Verification items for the finished model (mm, model axes). A direction names the side the tool comes from. Coordinates: 2 decimals unless noted, no trailing zeros. Loops run counter-clockwise (first coordinate to the right, second up) from the corner with the lowest first, then second, coordinate; pieces in that order, holes last. Notation, with made-up numbers: (82, 31.25) - (126, 31.25) arc R10 cw to (126, 35.25) - close; hole circle Ø4 at (-21.5, -19). An arc over 180 degrees is marked (long way). Answer as CSV lines item,"result". Start each with the question number.
1. Gauge pin test, flat ends, axial feed: P1, Ø3, axis at x = 0, z = 15, coming from the +Y side; P2, Ø4, axis at y = 4, z = 26.5, coming from the -X side; P3, Ø4, axis at x = 0, z = 5, coming from the +Y side. Record the tip position at first contact, or that the pin passes through.
2. Release check for a two-part mould opening along Z. For faces 1 (the flat face through (-0.1, 0.7, 30)), 2 (the flat face through (-0.1, 0.7, 0)), 3 (the flat face through (2.04, 1, 14.79)), 4 (the cylindrical face through (-0.24, 0.01, 13.14)) record: pulls with the +Z half, pulls with the -Z half, needs draft (parallel to the pull), parting line crosses it, or undercut.
3. Cross-section at C-C (x = 4). Enter the section's corners in (y, z) (3 decimals), plus the area to 3 significant figures.
4. Cross-section at B-B (y = 7.5). Enter the section's corners in (x, z).
5. Cross-section at A-A (z = 25). Enter the section's corners in (x, y), plus the area to 3 significant figures.
6. Material ranges on line 1 (Z direction, x = 3.65, y = 4) (3 decimals); line 2 (X direction, y = 3, z = 9); line 3 (Y direction, x = 4, z = 25), recorded low to high. Write a range as [from, to].
7. Cross-section at D-D (y = 4.75). State how many separate pieces and enclosed holes the cut face has, plus the area to 3 significant figures.
8. Set-up check for faces 5 (the flat face through (3, 7, 15)), 6 (the flat face through (-5, 1.8, 14.8)): record each of +Z, -Z, +X, -X, +Y, -Y from which the full face is reachable in a straight line by a thin tool's end or side.
```python
from build123d import *

# Parameters (mm, degrees)
BOSS_EXTRUDE1_DEPTH     = 30
SKETCH2_R               = 1.75
SKETCH2_R_2             = 2
SKETCH2_R_3             = 1.875
CUT_EXTRUDE2_DEPTH      = 9
CUT_EXTRUDE2_DEPTH_BACK = 3
SKETCH3_R               = 1.75
SKETCH3_R_2             = 1.875
SKETCH3_R_3             = 2
CUT_EXTRUDE3_DEPTH      = 10


with BuildPart() as part:
    # Sketch1 → Boss-Extrude1 (new body)
    with BuildSketch(Plane.XY):
        Polygon((3, 1), (-3, 1), (-3, 9), (-5, 9), (-5, -1), (5, -1), (5, 9), (3, 9), align=None)
    extrude(amount=BOSS_EXTRUDE1_DEPTH)

    # Sketch2 → Cut-Extrude2 (cut, two sides)
    with BuildSketch(Plane(origin=(-3, 0, 0), x_dir=(0, 0, -1), z_dir=(1, 0, 0))) as cut_extrude2_sk:
        with Locations((-25, 4)):
            Circle(SKETCH2_R)
        with Locations((-5, 4)):
            Circle(SKETCH2_R_2)
        with Locations((-15, 4)):
            Circle(SKETCH2_R_3)
    extrude(amount=CUT_EXTRUDE2_DEPTH, mode=Mode.SUBTRACT)
    extrude(cut_extrude2_sk.sketch, amount=-CUT_EXTRUDE2_DEPTH_BACK, mode=Mode.SUBTRACT)

    # Sketch3 → Cut-Extrude3 (cut)
    with BuildSketch(Plane(origin=(0, 1, 0), x_dir=(1, 0, 0), z_dir=(0, 1, 0))):
        with Locations((0, -5)):
            Circle(SKETCH3_R)
        with Locations((0, -15)):
            Circle(SKETCH3_R_2)
        with Locations((0, -25)):
            Circle(SKETCH3_R_3)
    extrude(amount=-CUT_EXTRUDE3_DEPTH, mode=Mode.SUBTRACT)


solid = part.part
```
Values follow:
1,P1,"passes through"
1,P2,"stops at x = -5"
1,P3,"stops at y = 1"
2,face 1,"pulls with the +Z half"
2,face 2,"pulls with the -Z half"
2,face 3,"needs draft"
2,face 4,"undercut"
3,outline,"(-1, 0) - (9, 0) - (9, 30) - (-1, 30) - close; hole circle Ø4 at (4, 5); hole circle Ø3.75 at (4, 15); hole circle Ø3.5 at (4, 25)"
3,area,"267 mm²"
4,outline,"(-5, 0) - (-3, 0) - (-3, 30) - (-5, 30) - close; (3, 0) - (5, 0) - (5, 30) - (3, 30) - close"
5,outline,"(-5, -1) - (-2, -1) - (-2, 1) - (-3, 1) - (-3, 2.25) - (-5, 2.25) - close; (-5, 5.75) - (-3, 5.75) - (-3, 9) - (-5, 9) - close; (2, -1) - (5, -1) - (5, 2.25) - (3, 2.25) - (3, 1) - (2, 1) - close; (3, 5.75) - (5, 5.75) - (5, 9) - (3, 9) - close"
5,area,"30.0 mm²"
6,line 1,"z = [0, 3], [7, 13.125], [16.875, 23.25], [26.75, 30]"
6,line 2,"x = [-5, -3], [3, 5]"
6,line 3,"y = [-1, 2.25], [5.75, 9]"
7,separate pieces,"8"
7,enclosed holes,"0"
7,area,"78.8 mm²"
8,face 5,"+Z, -Z, +Y"
8,face 6,"+Z, -Z, -X, +Y, -Y"
